Design review of the part built by this model. Coordinates are the model's own, in mm. Face numbers are marked on the shaded views. Coordinates: 2 decimals unless noted, no trailing zeros. Order: outer loops, then holes, each group sorted by start corner. A loop starts at its lowest first (then second) coordinate and runs counter-clockwise, first axis right, second up. Notation, with made-up numbers: M 24,83 L 28,83 A17 cw 28,110 Z; hole C 12.5,79 d9. An arc over 180 degrees is marked long. Answer as a JSON object with one key per item and string values.
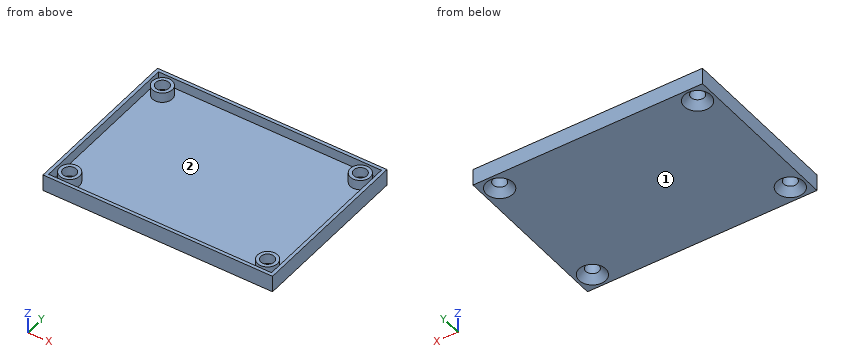
from build123d import *

# Parameters (mm, degrees)
F0_W     = 67
F0_H     = 48
F0_R     = 3
F1_DEPTH = 2
F0_R_2   = 2
F2_DEPTH = 5
F0_W_2   = 69
F0_H_2   = 50
F3_DEPTH = 5
F4_SIZE  = 2


with BuildPart() as f1:
    # F0 (on Top) → F1 (new body)
    with BuildSketch(Plane.XY):
        Rectangle(F0_W, F0_H)
        with Locations((-29.75, -20.25)):
            Circle(F0_R, mode=Mode.SUBTRACT)
        with Locations((29.75, -20.25)):
            Circle(F0_R, mode=Mode.SUBTRACT)
        with Locations((-29.75, 20.25)):
            Circle(F0_R, mode=Mode.SUBTRACT)
        with Locations((29.75, 20.25)):
            Circle(F0_R, mode=Mode.SUBTRACT)
    extrude(amount=F1_DEPTH)

    # F0 (on Top) → F2 (join)
    with BuildSketch(Plane.XY):
        with Locations((-29.75, 20.25)):
            Circle(F0_R)
        with Locations((-29.75, 20.25)):
            Circle(F0_R_2, mode=Mode.SUBTRACT)
        with Locations((29.75, 20.25)):
            Circle(F0_R)
        with Locations((29.75, 20.25)):
            Circle(F0_R_2, mode=Mode.SUBTRACT)
        with Locations((29.75, -20.25)):
            Circle(F0_R)
        with Locations((29.75, -20.25)):
            Circle(F0_R_2, mode=Mode.SUBTRACT)
        with Locations((-29.75, -20.25)):
            Circle(F0_R)
        with Locations((-29.75, -20.25)):
            Circle(F0_R_2, mode=Mode.SUBTRACT)
    extrude(amount=F2_DEPTH)

    # F0 (on Top) → F3 (join)
    with BuildSketch(Plane.XY):
        Rectangle(F0_W_2, F0_H_2)
        Rectangle(F0_W, F0_H, mode=Mode.SUBTRACT)
    extrude(amount=F3_DEPTH)

    # F4
    f4_edges = [f1.edges().sort_by_distance(p)[0] for p in [
        (27.75, -20.25, 0),
        (27.75, 20.25, 0),
        (-31.75, 20.25, 0),
        (-31.75, -20.25, 0),
    ]]
    chamfer(f4_edges, length=F4_SIZE)


solid = f1.part
1) Add section D-D (x = -15). State the section outline as (y, z) points, and give its area (3 significant figures).
Taken from the geometry:
{"outline": "M -25,0 L 25,0 L 25,5 L 24,5 L 24,2 L -24,2 L -24,5 L -25,5 Z", "area": "106 mm2"}
2) Add section B-B (y = 20.25). State the section outline as (x, z) points, and give its area (3 significant figures).
Taken from the geometry:
{"outline": "M -34.5,0 L -33.75,0 L -31.75,2 L -31.75,5 L -32.75,5 L -32.75,2 L -33.5,2 L -33.5,5 L -34.5,5 Z; M -27.75,2 L -25.75,0 L 25.75,0 L 27.75,2 L 27.75,5 L 26.75,5 L 26.75,2 L -26.75,2 L -26.75,5 L -27.75,5 Z; M 31.75,2 L 33.75,0 L 34.5,0 L 34.5,5 L 33.5,5 L 33.5,2 L 32.75,2 L 32.75,5 L 31.75,5 Z", "area": "132 mm2"}
3) Insertion check: pin 1 Ø6 at (x, y) = (25.5, -0.5) entering from +Z; pin 2 Ø5 at (x, y) = (-29.75, -20.25) entering from -Z. Each pin has a flat end and moves straight along its axis. Give the tip position at first contact, or say it passes through.
Taken from the geometry:
{"pin 1": "stops at z = 2", "pin 2": "stops at z = 1.5"}
4) Add section C-C (y = -4.5). State the section outline as (x, z) points, and give its area (3 significant figures).
Taken from the geometry:
{"outline": "M -34.5,0 L 34.5,0 L 34.5,5 L 33.5,5 L 33.5,2 L -33.5,2 L -33.5,5 L -34.5,5 Z", "area": "144 mm2"}
5) Mouldability with a two-part tool opening along X and no side actions: class the marked faces 1 and 2 as released by +X, released by -X, zero draft, split by the parting line, or undercut.
Taken from the geometry:
{"face 1": "zero draft", "face 2": "undercut"}
6) Add section A-A (x = 29.75). State the section outline as (y, z) points.
Taken from the geometry:
{"outline": "M -25,0 L -24.25,0 L -22.25,2 L -22.25,5 L -23.25,5 L -23.25,2 L -24,2 L -24,5 L -25,5 Z; M -18.25,2 L -16.25,0 L 16.25,0 L 18.25,2 L 18.25,5 L 17.25,5 L 17.25,2 L -17.25,2 L -17.25,5 L -18.25,5 Z; M 22.25,2 L 24.25,0 L 25,0 L 25,5 L 24,5 L 24,2 L 23.25,2 L 23.25,5 L 22.25,5 Z"}
7) To check wall thickness, follow L1, parallel to X at y = 20, z = 3.65; L2, parallel to Y at x = 29.75, z = 3; L3, parallel to Y at x = -23, z = 4.65. State the ranges of each line that lie inside material, in increasing order.
Taken from the geometry:
{"L1": "x = -34.5 to -33.5, -32.74 to -31.73, -27.77 to -26.76, 26.76 to 27.77, 31.73 to 32.74, 33.5 to 34.5", "L2": "y = -25 to -24, -23.25 to -22.25, -18.25 to -17.25, 17.25 to 18.25, 22.25 to 23.25, 24 to 25", "L3": "y = -25 to -24, 24 to 25"}
